Build history of the part. All positions in model axes, mm. Give positions to 0.01 mm unless a question says otherwise; leave off trailing zeros. Order: outer loops, then holes, each group sorted by start corner. A loop starts at its lowest first (then second) coordinate and runs counter-clockwise, first axis right, second up. Notation, with made-up numbers: (75.25, 58) - (122.25, 58) arc R11 cw to (122.25, 74) - close; hole circle Ø5 at (45.5, 9.25). An arc over 180 degrees is marked (long way). Use a Markdown table: item, result.
from build123d import *

# Parameters (mm, degrees)
F0_R     = 11.049
F1_DEPTH = 6.35


with BuildPart() as f1:
    # F0 (on Top) → F1 (new body)
    with BuildSketch(Plane.XY):
        with BuildLine():
            ThreePointArc((0, 16.530267), (-9.878282, 20.621985), (-13.97, 30.500267))
            ThreePointArc((-13.97, 30.500267), (-17.499453, 0.425585), (-13.97, -29.649097))
            ThreePointArc((-13.97, -29.649097), (-9.878282, -19.770816), (0, -15.679097))
            Line((0, -15.679097), (0, -13.97))
            ThreePointArc((0, -13.97), (-13.97, 0), (0, 13.97))
            Line((0, 13.97), (0, 16.530267))
        make_face()
        with BuildLine():
            ThreePointArc((13.97, 30.500267), (10.194271, 40.052111), (0.908048, 44.440724))
            ThreePointArc((0.908048, 44.440724), (0, 44.45), (-0.908048, 44.440724))
            ThreePointArc((-0.908048, 44.440724), (-10.194271, 40.052111), (-13.97, 30.500267))
            ThreePointArc((-13.97, 30.500267), (-9.878282, 20.621985), (0, 16.530267))
            ThreePointArc((0, 16.530267), (9.878282, 20.621985), (13.97, 30.500267))
        make_face()
        with Locations((0, 30.500267)):
            Circle(F0_R, mode=Mode.SUBTRACT)
        with BuildLine():
            ThreePointArc((13.97, -29.649097), (18.582887, 0.425585), (13.97, 30.500267))
            ThreePointArc((13.97, 30.500267), (9.878282, 20.621985), (0, 16.530267))
            Line((0, 16.530267), (0, 13.97))
            ThreePointArc((0, 13.97), (9.878282, 9.878282), (13.97, 0))
            ThreePointArc((13.97, 0), (9.878282, -9.878282), (0, -13.97))
            Line((0, -13.97), (0, -15.679097))
            ThreePointArc((0, -15.679097), (9.878282, -19.770816), (13.97, -29.649097))
        make_face()
        with BuildLine():
            Line((0, 11.049), (0, 13.97))
            ThreePointArc((0, 13.97), (-13.97, 0), (0, -13.97))
            Line((0, -13.97), (0, -11.049))
            ThreePointArc((0, -11.049), (-11.049, 0), (0, 11.049))
        make_face()
        with BuildLine():
            ThreePointArc((13.97, 0), (9.878282, 9.878282), (0, 13.97))
            Line((0, 13.97), (0, 11.049))
            ThreePointArc((0, 11.049), (7.812823, 7.812823), (11.049, 0))
            ThreePointArc((11.049, 0), (7.812823, -7.812823), (0, -11.049))
            Line((0, -11.049), (0, -13.97))
            ThreePointArc((0, -13.97), (9.878282, -9.878282), (13.97, 0))
        make_face()
        with BuildLine():
            ThreePointArc((-13.97, -29.649097), (0, -43.619097), (13.97, -29.649097))
            ThreePointArc((13.97, -29.649097), (9.878282, -19.770816), (0, -15.679097))
            ThreePointArc((0, -15.679097), (-9.878282, -19.770816), (-13.97, -29.649097))
        make_face()
        with Locations((0, -29.649097)):
            Circle(F0_R, mode=Mode.SUBTRACT)
    extrude(amount=F1_DEPTH)


solid = f1.part
1) Slice it at D-D (y = 6.5). Write the cut outline in (x, z), and give its area (3 significant figures).
Computed:
| item | result |
|---|---|
| outline | (-17.36, 0) - (-8.93, 0) - (-8.93, 6.35) - (-17.36, 6.35) - close; (8.93, 0) - (18.4, 0) - (18.4, 6.35) - (8.93, 6.35) - close |
| area | 114 mm² |
2) Slice it at B-B (x = 2). Write the cut outline in (y, z), and give its area (3 significant figures).
Computed:
| item | result |
|---|---|
| outline | (-43.48, 0) - (-40.52, 0) - (-40.52, 6.35) - (-43.48, 6.35) - close; (-18.78, 0) - (-10.87, 0) - (-10.87, 6.35) - (-18.78, 6.35) - close; (10.87, 0) - (19.63, 0) - (19.63, 6.35) - (10.87, 6.35) - close; (41.37, 0) - (44.33, 0) - (44.33, 6.35) - (41.37, 6.35) - close |
| area | 144 mm² |
3) Slice it at A-A (z = 4). Write the cut outline in (x, y).
Computed:
| item | result |
|---|---|
| outline | (-13.97, -29.65) arc R13.97 ccw to (13.97, -29.65) arc R100.35 ccw to (13.97, 30.5) arc R13.97 ccw to (0.91, 44.44) arc R44.45 ccw to (-0.91, 44.44) arc R13.97 ccw to (-13.97, 30.5) arc R129.9 ccw to start; hole circle Ø22.1 at (0, -29.65); hole circle Ø22.1 at (0, 30.5); hole (0, 11.05) arc R11.05 ccw (long way) to (11.05, 0) arc R11.05 ccw to start |
4) Wall check: line 1 (Y direction, x = -9.5, z = 3.25); line 2 (Y direction, x = -3, z = 4.5); line 3 (X direction, y = -27.5, z = 5.25). Give the ranges that are in metal, low to high. Write a range as from..to.
Computed:
| item | result |
|---|---|
| line 1 | y = -39.89..-35.29, -24.01..-5.64, 5.64..24.86, 36.14..40.74 |
| line 2 | y = -43.29..-40.28, -19.02..-10.63, 10.63..19.87, 41.13..44.14 |
| line 3 | x = -14.46..-10.84, 10.84..14.62 |
5) Two-plate mould, pull along Y, no slides. Class faces 1 (the cylindrical face through (-0.307, -43.616, 3.131)), 2 (the cylindrical face through (-1.438, -18.694, 3.131)), 3 (the cylindrical face through (18.58, 0, 3.13)), 4 (the cylindrical face through (-2.395, 19.714, 3.131)): +Y half, -Y half, draft (parallel to the pull), parting line (faces both ways), or undercut.
Computed:
| item | result |
|---|---|
| face 1 | -Y half |
| face 2 | undercut |
| face 3 | parting line |
| face 4 | undercut |
6) Pin check, flat tips, straight feed: P1, Ø20, axis at x = 0, y = 30.5, coming from the +Z side; P2, Ø1.5, axis at y = -11.5, z = 5, coming from the -X side. Stop position of each tip, or through.
Computed:
| item | result |
|---|---|
| P1 | passes through |
| P2 | stops at x = -17.02 |
7) Slice it at C-C (y = -4). Write the cut outline in (x, z), and give its area (3 significant figures).
Computed:
| item | result |
|---|---|
| outline | (-17.42, 0) - (-10.3, 0) - (-10.3, 6.35) - (-17.42, 6.35) - close; (10.3, 0) - (18.49, 0) - (18.49, 6.35) - (10.3, 6.35) - close |
| area | 97.2 mm² |
